Build history of the part. All positions in model axes, mm. A direction names the side the tool comes from. Give positions to 0.01 mm unless a question says otherwise; leave off trailing zeros. Loops run counter-clockwise (first coordinate to the right, second up) from the corner with the lowest first, then second, coordinate; pieces in that order, holes last. Notation, with made-up numbers: (-9.75, 81) - (44.25, 81) arc R18 ccw to (44.25, 96) - close; hole circle Ø3 at (59, 29.5). An arc over 180 degrees is marked (long way). Return JSON: item names as keys, results as strings. Group by question number.
1) 3-axis set-ups, long thin cutter, end or side, ignore diameter. For faces 4 (the face through (37, 0, 0)), 5 (the face through (45, -1, -2)): which of +Z, -Z, +X, -X, +Y, -Y reach the whole face in a straight line?
2) Mould opens along Z. For faces 1 (the face through (2, -1, 2)), 2 (the face through (23.2, -0.83, 3.76)), 3 (the face through (41.1, 1.4, -1.9)) say: released by +Z, released by -Z, zero draft, split by the parting line, or undercut.
3) Drill centre lines: probe 1 along Y at (x, z) = (6, -2.25) (3 decimals); probe 2 along Y at (x, z) = (39, -2); probe 3 along X at (y, z) = (0, 1.5). Where is each one in solid material? Low to high. Write a range as from..to.
4) Slice it at A-A (x = 39). List the corners of the cut face in (y, z), and give its area (3 significant figures).
5) Drop flat-ended pins along their axis: pin 1 (4 mm diameter, centred on y = -0.5, z = 0, fed in from +X); pin 2 (1.4 mm diameter, centred on y = 0, z = 0.5, fed in from -X); pin 3 (1.5 mm diameter, centred on x = 35, y = 1, fed in from -Z). Give the stop position or say it passes through.
6) Slice it at C-C (z = 3.25). List the corners of the cut face in (x, y).
7) Slice it at B-B (x = 22.5). List the corners of the cut face in (y, z), and give its area (3 significant figures).
Autodesk Inventor part; units mm, degrees
ref_plane "YZ Plane" through (0, 0, 0) normal (1, 0, 0) x (0, 1, 0)
ref_plane "XZ Plane" through (0, 0, 0) normal (0, 1, 0) x (-1, 0, 0)
ref_plane "XY Plane" through (0, 0, 0) normal (0, 0, 1) x (1, 0, 0)
sketch "Sketch1" plane through (0, 0, 0) normal (1, 0, 0) x (0, 1, 0)
  circle A0 centre (0, 0) radius 3.85
  dimension "d0" = 7.7
extrude "Extrusion1" add sketch "Sketch1" along normal blind 5
sketch "Sketch2" plane through (5, 0, 0) normal (1, 0, 0) x (0, 0, -1)
  circle A0 centre (0, 0) radius 3.85
  dimension "d3" = 7.7
extrude "Extrusion2" add sketch "Sketch2" along normal blind 18.5
sketch "Sketch5" plane through (0, 0, 0) normal (-1, 0, 0) x (0, 0, 1)
  circle A0 centre (0, 0) radius 2.4
  line L0 (0, 0) -> (-2.4, 0)
  line L1 (-2.4, 0) -> (-2.4, 2.4)
  line L2 (-2.4, 2.4) -> (0, 2.4)
  line L3 (0, 2.4) -> (0, 0)
  line L4 (-2.4, 2.4) -> (2.4, 2.4)
  line L5 (2.4, 2.4) -> (2.4, -2.4)
  line L6 (2.4, -2.4) -> (-2.4, -2.4)
  line L7 (-2.4, -2.4) -> (-2.4, 2.4)
  line L8 (-2.4, 2.4) -> (2.4, 0)
  line L9 (-2.4, -2.4) -> (2.4, 0)
  line L10 (-2.4, 0) -> (2.4, 2.4)
  line L11 (-2.4, 0) -> (2.4, -2.4)
  line L12 (0, 2.4) -> (2.4, -2.4)
  line L13 (-2.4, -2.4) -> (0, 2.4)
  line L14 (-2.4, 2.4) -> (0, -2.4)
  line L15 (0, -2.4) -> (2.4, 2.4)
  point P0 (1.44, -0.48)
  point P1 (1.44, 0.48)
  point P2 (0.48, 1.44)
  point P3 (-0.48, 1.44)
  point P4 (-1.44, 0.48)
  point P5 (-1.44, -0.48)
  point P6 (-0.48, -1.44)
  point P7 (0.48, -1.44)
  dimension "d23" = 4.8
extrude "Extrusion5" cut sketch "Sketch5" against normal blind 10 contours L9 L12 L15 L8 | L15 L8 L12 L10 A0 | A0 L10 L15 | L12 L11 A0 | A0 L11 L15 L9 L12 | L15 L12 L8 | L9 L15 L12 | L12 L10 L3 | L3 L8 L13 | L14 L9 L11 L15 | L12 L15 L9 L11 L14 L0 L3 L8 | L8 L10 L12 | L15 L11 L9 | L8 L13 L10 L14 A0 | A0 L14 L8 | L10 L13 L8 | L3 L0 L13 L10 | L9 L13 A0 | A0 L13 L11 L14 L9 | L14 L11 L9 | L10 L14 L0 | L0 L13 L11 | L13 L14 L10 | L11 L13 L14
sketch "Sketch7" plane through (0, 0, 0) normal (-1, 0, 0) x (0, 0, 1)
  circle A0 centre (0, 0) radius 3.85
extrude "Extrusion7" cut sketch "Sketch7" against normal blind 2
mirror "Mirror1" about plane through (23.5, 0, 0) normal (1, 0, 0)
properties part number "gear_shaft"
Results:
{
 "1": {"face 4": "+X", "face 5": "+Z, -Z, +X, +Y, -Y"},
 "2": {"face 1": "zero draft", "face 2": "split by the parting line", "face 3": "undercut"},
 "3": {"probe 1": "-3.124..-2.325, -2.1..-0.075, 0.075..2.1, 2.325..3.124", "probe 2": "-3.29..-2.2, -1.6..-0.2, 0.2..1.6, 2.2..3.29", "probe 3": "10..37"},
 "4": {"outline": "circle Ø7.7 at (0, 0); hole (-2.4, -2.4) - (-0.48, -1.44) - (0, -2.4) - (0.48, -1.44) - (2.4, -2.4) - (1.44, -0.48) - (2.4, 0) - (1.44, 0.48) - (2.4, 2.4) - (0.48, 1.44) - (0, 2.4) - (-0.48, 1.44) - (-2.4, 2.4) - (-1.44, 0.48) - (-2.4, 0) - (-1.44, -0.48) - close", "area": "32.7 mm2"},
 "5": {"pin 1": "x = 45", "pin 2": "x = 10", "pin 3": "z = -3.84"},
 "6": {"outline": "(2, -2.06) - (45, -2.06) - (45, 2.06) - (2, 2.06) - close"},
 "7": {"outline": "circle Ø7.7 at (0, 0)", "area": "46.6 mm2"}
}
